Verification items for the finished model (mm, model axes). Face numbers are marked on the shaded views. A direction names the side the tool comes from. Give positions to 0.01 mm unless a question says otherwise; leave off trailing zeros. Order: outer loops, then holes, each group sorted by start corner. A loop starts at its lowest first (then second) coordinate and runs counter-clockwise, first axis right, second up. Notation, with made-up numbers: (22, 36.5) -> (41, 36.5) arc R19 cw to (41, 59.5) -> close; hole circle Ø1 at (83, 5.25). An arc over 180 degrees is marked (long way). One line per question, with ' | ' between items. Start each with the question number.
Q1. Section check C-C on x = -6.25. Record the cut outline in (y, z), plus the area to 3 significant figures.
Q2. Go/stop test with flat-tipped pins: pin 1 (2 mm diameter, centred on x = 6, y = 1.5, fed in from -Z); pin 2 (2.5 mm diameter, centred on x = 1, y = 3, fed in from +Z); pin 3 (0.8 mm diameter, centred on y = 2, z = 2.5, fed in from -X). Record where each tip stops, or that it passes through.
Q3. Section check B-B on z = 2.5. Record the cut outline in (x, y).
Q4. Section check A-A on z = -9.5. Record the cut outline in (x, y) (3 decimals).
Q5. Access from +Z, -Z, +X, -X, +Y, -Y to the whole of each face (thin tool, end or side, straight path). Record for the marked faces 1, 2, 3 and 4.
Q6. Material ranges on probe 1 along Z at (x, y) = (3, 1.75); probe 2 along Z at (x, y) = (-3, 2.4); probe 3 along X at (y, z) = (2.5, -8.5), recorded low to high. Write a range as [from, to].
from build123d import *

# Parameters (mm, degrees)
SKETCH1_W           = 17.5
SKETCH1_H           = 21
BOSS_EXTRUDE1_DEPTH = 1.2
FILLET1_R           = 1.88
SKETCH2_W           = 12
SKETCH2_H           = 11
BOSS_EXTRUDE2_DEPTH = 2
FILLET2_R           = 0.5
SKETCH3_W           = 8.94
SKETCH3_H           = 7.3
BOSS_EXTRUDE3_DEPTH = 3.21
FILLET3_R           = 1.25
CUT_EXTRUDE1_DEPTH  = 5


with BuildPart() as part:
    # Sketch1 → Boss-Extrude1 (new body)
    with BuildSketch(Plane(origin=(0, 0, 0), x_dir=(1, 0, 0), z_dir=(0, 1, 0))):
        Rectangle(SKETCH1_W, SKETCH1_H)
    extrude(amount=BOSS_EXTRUDE1_DEPTH)

    # Fillet1
    fillet1_edges = [part.edges().sort_by_distance(p)[0] for p in [
        (-8.75, 0.6, -10.5),
        (8.75, 0.6, -10.5),
        (8.75, 0.6, 10.5),
        (-8.75, 0.6, 10.5),
    ]]
    fillet(fillet1_edges, radius=FILLET1_R)

    # Sketch2 → Boss-Extrude2 (add)
    with BuildSketch(Plane(origin=(0, 1.2, 0), x_dir=(1, 0, 0), z_dir=(0, 1, 0))):
        with Locations((0, -2)):
            Rectangle(SKETCH2_W, SKETCH2_H)
    extrude(amount=BOSS_EXTRUDE2_DEPTH)

    # Fillet2
    fillet2_edges = [part.edges().sort_by_distance(p)[0] for p in [
        (-6, 2.2, -3.5),
        (-6, 2.2, 7.5),
        (6, 2.2, 7.5),
        (6, 2.2, -3.5),
        (-6, 3.2, 2),
        (0, 3.2, 7.5),
        (6, 3.2, 2),
        (0, 3.2, -3.5),
    ]]
    fillet(fillet2_edges, radius=FILLET2_R)

    # Sketch3 → Boss-Extrude3 (add)
    with BuildSketch(Plane(origin=(0, 1.2, 0), x_dir=(1, 0, 0), z_dir=(0, 1, 0))):
        with Locations((0, 7.85)):
            Rectangle(SKETCH3_W, SKETCH3_H)
    extrude(amount=BOSS_EXTRUDE3_DEPTH)

    # Fillet3
    fillet3_edges = [part.edges().sort_by_distance(p)[0] for p in [
        (-4.47, 1.2, -11),
        (4.47, 1.2, -11),
        (-4.47, 4.41, -7.85),
        (4.47, 4.41, -7.85),
    ]]
    fillet(fillet3_edges, radius=FILLET3_R)

    # Sketch4 → Cut-Extrude1 (cut)
    with BuildSketch(Plane(origin=(0, 0, -11.5), x_dir=(-1, 0, 0), z_dir=(0, 0, -1))):
        with BuildLine():
            Line((-3.25, 3.805), (3.25, 3.805))
            ThreePointArc((3.25, 3.805), (4.25, 2.805), (3.25, 1.805))
            Line((3.25, 1.805), (-3.25, 1.805))
            ThreePointArc((-3.25, 1.805), (-4.25, 2.805), (-3.25, 3.805))
        make_face()
        with BuildLine():
            Line((-2.5, 3.305), (2.5, 3.305))
            ThreePointArc((2.5, 3.305), (3, 2.805), (2.5, 2.305))
            Line((2.5, 2.305), (-2.5, 2.305))
            ThreePointArc((-2.5, 2.305), (-3, 2.805), (-2.5, 3.305))
        make_face(mode=Mode.SUBTRACT)
    extrude(amount=-CUT_EXTRUDE1_DEPTH, mode=Mode.SUBTRACT)


solid = part.part
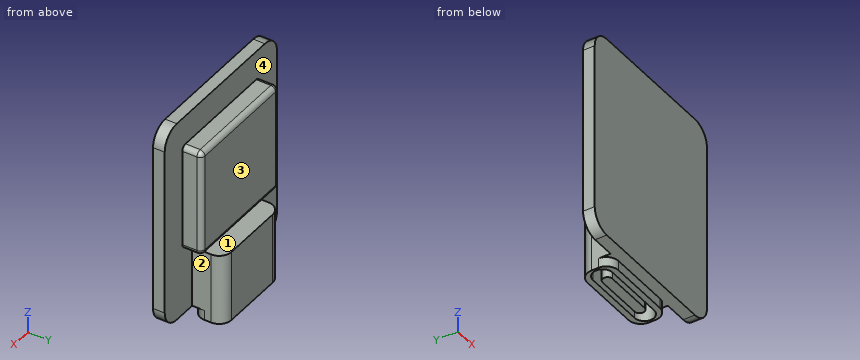
Filled in:
1) outline: (0, -10.5) -> (1.2, -10.5) -> (1.2, 10.5) -> (0, 10.5) -> close | area: 25.2 mm²
2) pin 1: z = -10.5 | pin 2: z = 7.5 | pin 3: x = -6
3) outline: (-8.75, 0) -> (8.75, 0) -> (8.75, 1.2) -> (6, 1.2) -> (6, 2.7) arc R0.5 ccw to (5.5, 3.2) -> (-5.5, 3.2) arc R0.5 ccw to (-6, 2.7) -> (-6, 1.2) -> (-8.75, 1.2) -> close
4) outline: (-8.531, 0) -> (8.531, 0) -> (8.531, 1.2) -> (4.47, 1.2) -> (4.47, 3.16) arc R1.25 ccw to (3.22, 4.41) -> (-3.22, 4.41) arc R1.25 ccw to (-4.47, 3.16) -> (-4.47, 1.2) -> (-8.531, 1.2) -> close; (-2.5, 2.305) -> (2.5, 2.305) arc R0.5 ccw to (2.5, 3.305) -> (-2.5, 3.305) arc R0.5 ccw to start; hole (-3.25, 1.805) -> (3.25, 1.805) arc R1 ccw to (3.25, 3.805) -> (-3.25, 3.805) arc R1 ccw to start
5) face 1: +X, -X, +Y | face 2: -Z, +X, +Y | face 3: +Z, +X, -X, +Y | face 4: +Y
6) probe 1: [-11.5, -4.2], [-3.5, 7.5] | probe 2: [-6.5, -4.2], [-3.5, 7.5] | probe 3: [-4.47, -4.2], [-2.9, 2.9], [4.2, 4.47]
